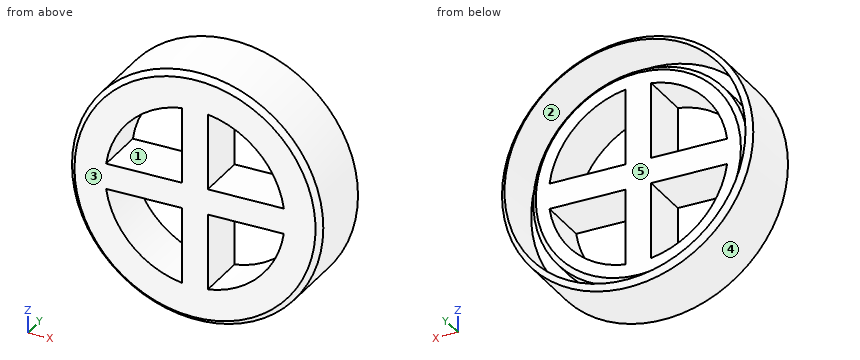
```python
from build123d import *

# Parameters (mm, degrees)
F3_DEPTH = 25
F4_SIZE  = 0.99999


# Not quite as in the source:
# - a fillet or chamfer is up to 0.001 mm smaller than in the source, because OpenCascade refuses the exact size


with BuildPart() as f1:
    # F0 (on Top) → F1 (revolve)
    with BuildSketch(Plane.XY):
        Polygon((-24.5, 15), (-24.5, 0), (0, 0), (0, 10), (-21, 10), (-21, 5), (-23.5, 5), (-23.5, 15), align=None)
    revolve(axis=Axis((0, 1.7348257825, 0), (0, 1, 0)))

    # F2 (on face) → F3 (cut)
    with BuildSketch(Plane(origin=(0, 10, 0), x_dir=(-1, 0, 0), z_dir=(0, 1, 0))):
        with BuildLine():
            Line((-2.5, -2.5), (-17.3205080757, -2.5))
            ThreePointArc((-17.3205080757, -2.5), (-12.3743686708, -12.3743686708), (-2.5, -17.3205080757))
            Line((-2.5, -17.3205080757), (-2.5, -2.5))
        make_face()
        with BuildLine():
            ThreePointArc((17.3205080757, 2.5), (12.3743686708, 12.3743686708), (2.5, 17.3205080757))
            Line((2.5, 17.3205080757), (2.5, 2.5))
            Line((2.5, 2.5), (17.3205080757, 2.5))
        make_face()
        with BuildLine():
            Line((-2.5, 2.5), (-2.5, 17.3205080757))
            ThreePointArc((-2.5, 17.3205080757), (-12.3743686708, 12.3743686708), (-17.3205080757, 2.5))
            Line((-17.3205080757, 2.5), (-2.5, 2.5))
        make_face()
        with BuildLine():
            Line((17.3205080757, -2.5), (2.5, -2.5))
            Line((2.5, -2.5), (2.5, -17.3205080757))
            ThreePointArc((2.5, -17.3205080757), (12.3743686708, -12.3743686708), (17.3205080757, -2.5))
        make_face()
    extrude(amount=-F3_DEPTH, mode=Mode.SUBTRACT)

    # F4 (size 1 in the source; OpenCascade refuses exactly that, so slightly less here)
    f4_edges = [f1.edges().sort_by_distance(p)[0] for p in [
        (24.5, 0, 0),
        (24.5, 15, 0),
        (21, 10, 0),
    ]]
    chamfer(f4_edges, length=F4_SIZE)


solid = f1.part
```
Check sheet for the modelled part. Datum: model origin and axes. Units: mm. Face numbers are marked on the shaded views. A direction names the side the tool comes from. Round coordinates to 2 decimals unless told otherwise and drop trailing zeros. Loops run counter-clockwise (first coordinate to the right, second up) from the corner with the lowest first, then second, coordinate; pieces in that order, holes last. Notation, with made-up numbers: (89.25, 12.25) - (146.25, 12.25) arc R15 ccw to (146.25, 31.25) - close; hole circle Ø2 at (68, 80). An arc over 180 degrees is marked (long way). Answer as a JSON object with one key per item and string values. Group by question number.
Q1. Sectioned sample at D-D, the plane x = -16. Count the separate pieces of the cut face and the enclosed holes in it, plus the area to 3 significant figures.
Q2. Sectioned sample at A-A, the plane y = 11.5. Enter the section's corners in (x, z).
Q3. Set-up check for the marked faces 1 and 2: record each of +Z, -Z, +X, -X, +Y, -Y from which the full face is reachable in a straight line by a thin tool's end or side.
Q4. Mould release check, pull along Z, two halves, no side actions. Record for the marked faces 3, 4 and 5: released by +Z, released by -Z, zero draft, split by the parting line, or undercut.
Q5. Gauge pin test, flat ends, axial feed: P1, Ø8, axis at y = 3, z = 10, coming from the -X side; P2, Ø3, axis at y = 6.5, z = 10, coming from the +X side; P3, Ø8, axis at x = -13, y = 3, coming from the -Z side; P4, Ø6, axis at x = 14.5, z = -16, coming from the -Y side. Record the tip position at first contact, or that the pin passes through.
Q6. Scan lines: line 1 along Z through (x, y) = (0, 8.75); line 2 along X through (y, z) = (10.5, -0.5); line 3 along X through (y, z) = (6.5, -14). Record each from-to range of solid material in increasing order. Write a range as [from, to].
Solution:
{
 "1": {"separate pieces": "3", "enclosed holes": "0", "area": "252 mm²"},
 "2": {"outline": "circle Ø49 at (0, 0); hole circle Ø47 at (0, 0)"},
 "3": {"face 1": "+Y, -Y", "face 2": "+Y"},
 "4": {"face 3": "zero draft", "face 4": "split by the parting line", "face 5": "undercut"},
 "5": {"P1": "stops at x = -23.75", "P2": "stops at x = 22.98", "P3": "stops at z = -22.79", "P4": "stops at y = 0"},
 "6": {"line 1": "z = [-24.5, -23.5], [-21, 21], [23.5, 24.5]", "line 2": "x = [-24.49, -23.49], [23.49, 24.49]", "line 3": "x = [-20.11, -18.87], [-15.65, -10.5], [-2.5, 2.5], [10.5, 15.65], [18.87, 20.11]"}
}
